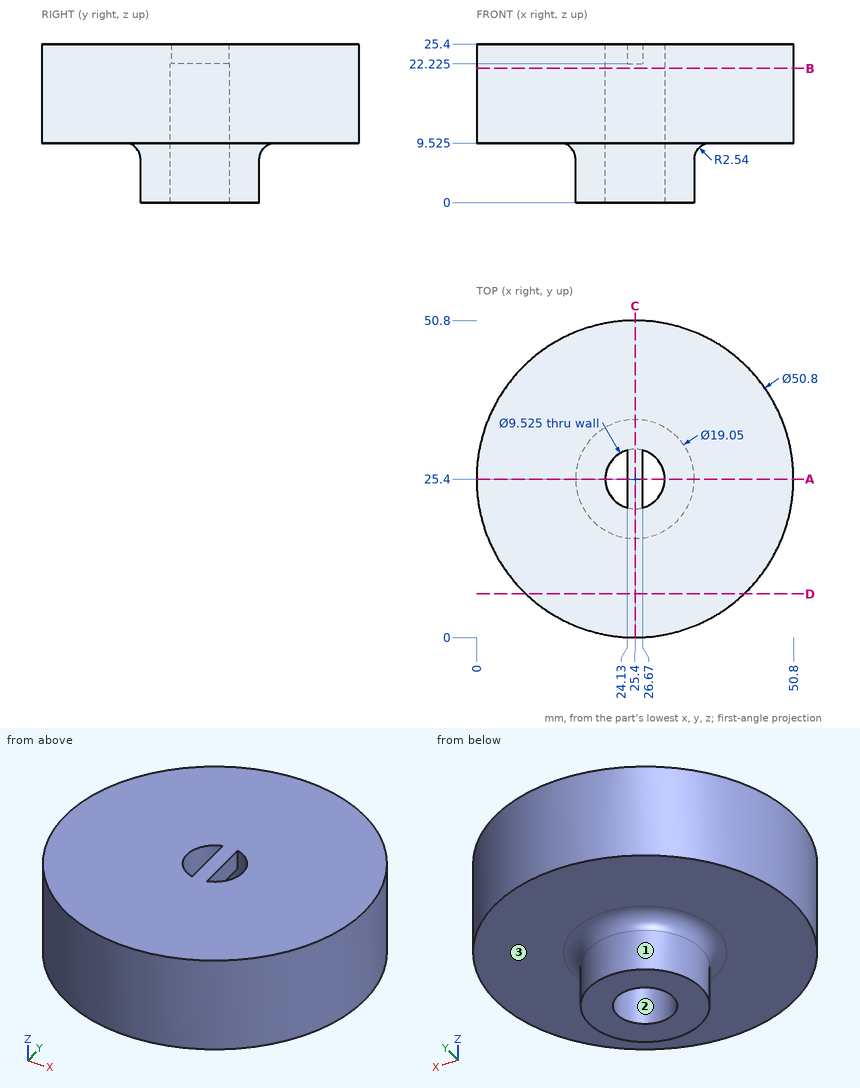
Job drawing, mm, ordinate dimensions from the low corner. One solid piece. Coordinates: 2 decimals unless noted, no trailing zeros. Write each loop counter-clockwise with the first axis right and the second up, starting at its lowest first coordinate (ties: lowest second). Pieces come first, ordered by that corner, then holes. Notation, with made-up numbers: (-33.5, -22) -> (22.5, -22) arc R15 ccw to (22.5, -6) -> close; hole circle Ø4 at (-25, 61). An arc over 180 degrees is marked (long way). Use CSV: the item, a comma, the result in double quotes. Start each with the question number.
Item 1: Drop flat-ended pins along their axis: P1, Ø10, axis at x = 32.5, y = 30, coming from the -Z side; P2, Ø2.5, axis at y = 27.5, z = 24, coming from the +X side; P3, Ø4, axis at x = 21.5, z = 8, coming from the +Y side; P4, Ø10, axis at y = 17, z = 13, coming from the -X side. Give the stop position or say it passes through.
Item 2: Band-saw the part on D-D, the plane y = 7. Write the cut outline in (x, z) (3 decimals).
Item 3: Two-plate mould, pull along Y, no slides. Class the marked faces 1, 2 and 3: +Y half, -Y half, draft (parallel to the pull), parting line (faces both ways), or undercut.
Item 4: Band-saw the part on B-B, the plane z = 21.5. Write the cut outline in (x, y) (1 decimal), plus the area to 3 significant figures.
Item 5: Wall check: probe 1 along Y at (x, z) = (25.4, 10.5); probe 2 along Z at (x, y) = (18.5, 42) (3 decimals); probe 3 along X at (y, z) = (28.5, 17). Give the ranges that are in metal, low to high.
Item 6: Band-saw the part on A-A, the plane y = 25.4. Write the cut outline in (x, z) (1 decimal).
Item 7: Band-saw the part on C-C, the plane x = 25.4. Write the cut outline in (y, z) (1 decimal), plus the area to 3 significant figures.
Response values:
1,P1,"stops at z = 0"
1,P2,"stops at x = 50.79"
1,P3,"stops at y = 50.67"
1,P4,"stops at x = 0.23"
2,outline,"(7.89, 9.525) -> (42.91, 9.525) -> (42.91, 25.4) -> (7.89, 25.4) -> close"
3,face 1,"parting line"
3,face 2,"undercut"
3,face 3,"draft"
4,outline,"circle Ø50.8 at (25.4, 25.4); hole circle Ø9.5 at (25.4, 25.4)"
4,area,"1,960 mm2"
5,probe 1,"y = 0 to 20.64, 30.16 to 50.8"
5,probe 2,"z = 9.525 to 25.4"
5,probe 3,"x = 0.19 to 21.78, 29.02 to 50.61"
6,outline,"(0, 9.5) -> (13.3, 9.5) arc R2.5 cw to (15.9, 7) -> (15.9, 0) -> (20.6, 0) -> (20.6, 25.4) -> (0, 25.4) -> close; (24.1, 22.2) -> (26.7, 22.2) -> (26.7, 25.4) -> (24.1, 25.4) -> close; (30.2, 0) -> (34.9, 0) -> (34.9, 7) arc R2.5 cw to (37.5, 9.5) -> (50.8, 9.5) -> (50.8, 25.4) -> (30.2, 25.4) -> close"
7,outline,"(0, 9.5) -> (13.3, 9.5) arc R2.5 cw to (15.9, 7) -> (15.9, 0) -> (20.6, 0) -> (20.6, 22.2) -> (30.2, 22.2) -> (30.2, 0) -> (34.9, 0) -> (34.9, 7) arc R2.5 cw to (37.5, 9.5) -> (50.8, 9.5) -> (50.8, 25.4) -> (0, 25.4) -> close"
7,area,"779 mm2"
